Design review of the part shown in the three views and the two pictorial views. Dimensions are in mm from the part's minimum x, y and z. Coordinates: 2 decimals unless noted, no trailing zeros. Write each loop counter-clockwise with the first axis right and the second up, starting at its lowest first coordinate (ties: lowest second). Pieces come first, ordered by that corner, then holes.
Q1. Take a section at A-A, the plane z = 2.15. Write out the cut boundary in (x, y).
Q2. For L1, parallel to Y at x = 82, z = 2.1; L2, parallel to X at y = 70.5, z = 2.2, list the stretches that pass through material, from the lowest coordinate up.
Q3. For pin 1 Ø1.4 at (x, z) = (98, 1) entering from +Y, flat-tipped, find the tip position at first contact; note if it passes through.
Q4. Take a section at B-B, the plane x = 108. Write out the cut boundary in (y, z).
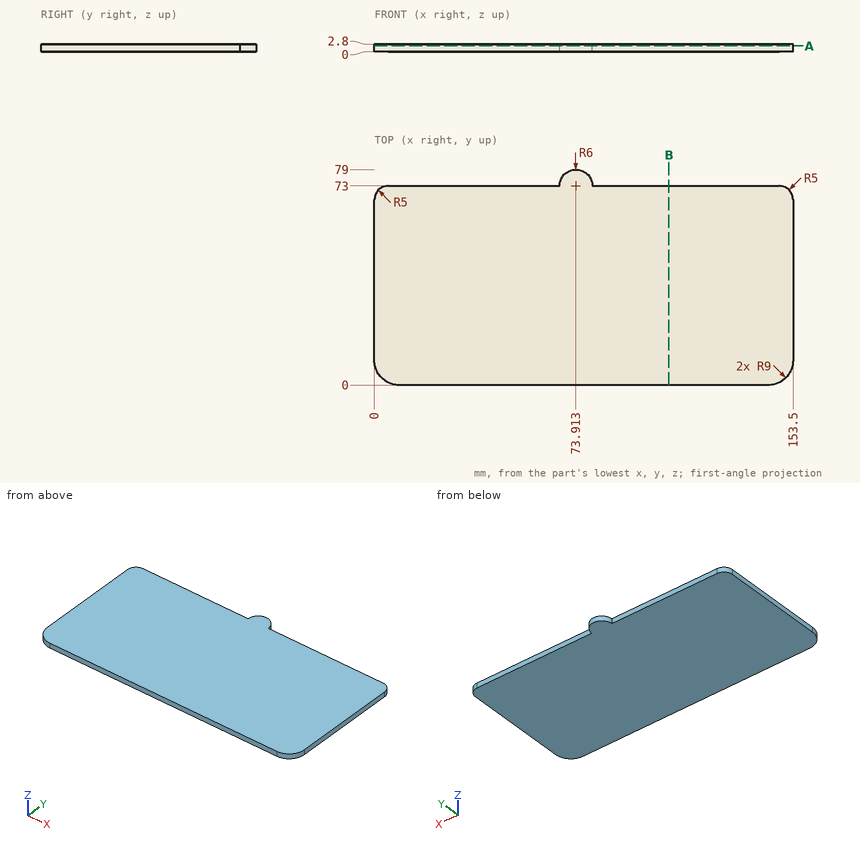
Responses:
1. outline: (0, 9) arc R9 ccw to (9, 0) - (144.5, 0) arc R9 ccw to (153.5, 9) - (153.5, 68) arc R5 ccw to (148.5, 73) - (79.91, 73) arc R6 ccw to (67.91, 73) - (5, 73) arc R5 ccw to (0, 68) - close
2. L1: y = 0 to 73
2. L2: x = 0.67 to 152.83
3. pin 1: stops at y = 73
4. outline: (0, 0) - (73, 0) - (73, 2.8) - (0, 2.8) - close
